Design review of the part built by this model. Coordinates are the model's own, in mm. Face numbers are marked on the shaded views. A direction names the side the tool comes from. Coordinates: 2 decimals unless noted, no trailing zeros. Loops run counter-clockwise (first coordinate to the right, second up) from the corner with the lowest first, then second, coordinate; pieces in that order, holes last. Notation, with made-up numbers: M -36,75.5 L 16,75.5 A9 cw 16,80.5 Z; hole C -23,20.5 d1. An arc over 180 degrees is marked long. Answer as a JSON object with one key per item and string values. Group by question number.
1. To check wall thickness, follow probe 1 along Y at (x, z) = (8.5, -3.75); probe 2 along Z at (x, y) = (0, 1.25); probe 3 along X at (y, z) = (-0.5, -0.5). State the ranges of each line that lie inside material, in increasing order.
2. Consider section B-B (x = 0). State the section outline as (y, z) points, then the cut area to 3 significant figures.
3. Draft analysis for pull direction Z (two halves, no side actions). For the marked faces 1, 2 and 3, state which applies: +Z half, -Z half, draft (parallel to the pull), parting line (faces both ways), or undercut.
4. Machinability: for the marked faces 4 and 5, which of the approach directions +Z, -Z, +X, -X, +Y, -Y give a long, thin tool a straight path to every point of the face, cutting with its end or side? Answer none if there is none.
5. Insertion check: pin 1 (1.5 mm diameter, centred on x = -2.5, y = 2, fed in from +Z); pin 2 (1.5 mm diameter, centred on y = -1, z = -3, fed in from -X); pin 3 (2 mm diameter, centred on x = 3.5, y = 1.5, fed in from -Z). Each pin has a flat end and moves straight along its axis. Give the tip position at first contact, or say it passes through.
6. Consider section C-C (y = 1.05). State the section outline as (x, z) points.
7. Consider section D-D (x = -7.75). State the section outline as (y, z) points.
8. Consider section A-A (z = 0). State the section outline as (x, y) points, then the cut area to 3 significant figures.
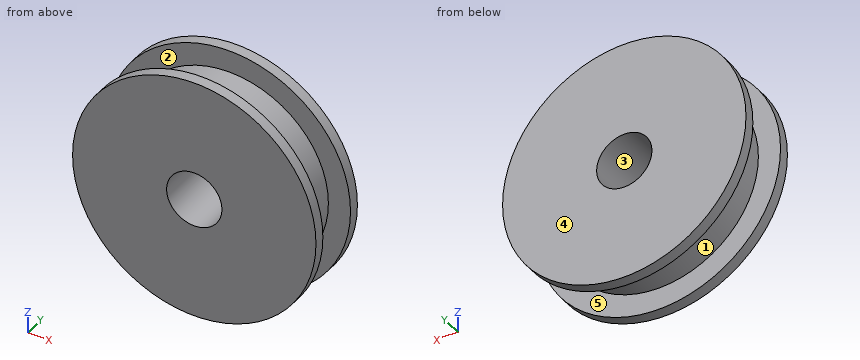
Autodesk Inventor part; units mm, degrees
ref_plane "YZ Plane" through (0, 0, 0) normal (1, 0, 0) x (0, 1, 0)
ref_plane "XZ Plane" through (0, 0, 0) normal (0, 1, 0) x (-1, 0, 0)
ref_plane "XY Plane" through (0, 0, 0) normal (0, 0, 1) x (1, 0, 0)
sketch "Sketch1" plane through (0, 0, 0) normal (0, 0, 1) x (1, 0, 0)
  line L0 (0, 3) -> (9, 3)
  line L1 (9, 3) -> (9, 0)
  line L2 (9, 0) -> (0, 0)
  line L3 (0, 0) -> (0, 3)
  line L4 (0, 3) -> (11, 3)
  line L5 (11, 3) -> (11, 2)
  line L6 (11, 2) -> (0, 2)
  line L7 (0, 2) -> (0, 3)
  point P0 (9, 2)
  dimension "d0" = 9
  dimension "d1" = 3
  dimension "d2" = 11
  dimension "d3" = 1
  dimension "d8" = 2
revolve "Revolution1" add sketch "Sketch1" angle 360 about axis through (0, 0, 0) along (0, 1, 0)
mirror "Mirror1" about plane through (0, 0, 0) normal (0, 1, 0) of "Revolution1"
sketch "Sketch2" plane through (0, -3, 0) normal (0, -1, 0) x (1, 0, 0)
  circle A0 centre (0, 0) radius 2.5
  point P0 (0, 0)
  dimension "d5" = 5
extrude "Extrusion1" cut sketch "Sketch2" against normal blind 10
properties part number "stove_pulley"
Findings below:
{
 "1": {"probe 1": "y = -3 to -2, 2 to 3", "probe 2": "z = -9 to -2.5, 2.5 to 9", "probe 3": "x = -8.99 to -2.45, 2.45 to 8.99"},
 "2": {"outline": "M -3,-11 L -2,-11 L -2,-9 L 2,-9 L 2,-11 L 3,-11 L 3,-2.5 L -3,-2.5 Z; M -3,2.5 L 3,2.5 L 3,11 L 2,11 L 2,9 L -2,9 L -2,11 L -3,11 Z", "area": "86.0 mm^2"},
 "3": {"face 1": "parting line", "face 2": "draft", "face 3": "undercut"},
 "4": {"face 4": "+Z, -Z, +X, -X, +Y", "face 5": "none"},
 "5": {"pin 1": "stops at z = 10.86", "pin 2": "stops at x = -8.71", "pin 3": "stops at z = -10.68"},
 "6": {"outline": "C 0,0 d18; hole C 0,0 d5"},
 "7": {"outline": "M -3,-7.81 L -2,-7.81 L -2,-4.58 L 2,-4.58 L 2,-7.81 L 3,-7.81 L 3,7.81 L 2,7.81 L 2,4.58 L -2,4.58 L -2,7.81 L -3,7.81 Z"},
 "8": {"outline": "M -11,-3 L -2.5,-3 L -2.5,3 L -11,3 L -11,2 L -9,2 L -9,-2 L -11,-2 Z; M 2.5,-3 L 11,-3 L 11,-2 L 9,-2 L 9,2 L 11,2 L 11,3 L 2.5,3 Z", "area": "86.0 mm^2"}
}
